from build123d import *

# Parameters (mm, degrees)
F3_R     = 2.291344539
F4_DEPTH = 2.5
F5_R     = 2.75
F6_DEPTH = 1


with BuildPart() as f1:
    # F0 (on Front) → F1 (revolve)
    with BuildSketch(Plane.XZ):
        with BuildLine():
            Line((-6, 0), (0, 0))
            Line((0, 0), (0, 12))
            add(Edge.make_bspline(
                [(0, 12), (-3.2266811418, 11.7082983458), (-6.2449243477, 6.1923159091), (-6.0526283931, 3.414490179), (-6, 0)],
                knots=[0, 0, 0, 0, 0.5139326164, 1, 1, 1, 1], degree=3))
        make_face()
    revolve(axis=Axis((0, 0, 6), (0, 0, 1)))

    # F3 (on offset) → F4 (join, symmetric)
    with BuildSketch(Plane.XY.offset(12)):
        Circle(F3_R)
    extrude(amount=F4_DEPTH, both=True)

    # F5 (on face) → F6 (join)
    with BuildSketch(Plane.XY.offset(14.5)):
        Circle(F5_R)
    extrude(amount=F6_DEPTH)


solid = f1.part
Can you work these out from the model? Positions are in its coordinate system, mm. Round coordinates to 2 decimals unless told otherwise and drop trailing zeros. Write each loop counter-clockwise with the first axis right and the second up, starting at its lowest first coordinate (ties: lowest second). Pieces come first, ordered by that corner, then holes. Notation, with made-up numbers: (-30.5, -8) -> (-13.5, -8) arc R8 cw to (-13.5, 2) -> close; hole circle Ø1 at (68.25, -11). An arc over 180 degrees is marked (long way). Use one line per item in the form item = value. Start each with the question number.
Q1. Imagine slicing it at A-A (z = 13). Please give me the cut outline in (x, y).
Q2. I'm going to push flat-ended pins straight in: P1, Ø3, axis at x = -2.5, y = -3.5, coming from the +Z side; P2, Ø4, axis at x = -4.5, y = 3.5, coming from the +Z side; P3, Ø4, axis at y = 1, z = 14, coming from the +X side. Where does each tip first touch, or does it pass through?
Q3. We'd pull the mould along Z, two halves only. Please class faces 1 (the face through (-0.596, -2.685, 14.993)), 2 (the face through (-2.29, 0.1, 12.9)), 3 (the face through (0, 0, 0)): +Z half, -Z half, draft (parallel to the pull), parting line (faces both ways), or undercut.
Q4. If I drill on probe 1 along X at (y, z) = (-0.5, 3.5); probe 2 along X at (y, z) = (1.75, 5.75); probe 3 along Z at (x, y) = (-4, -3.5), over which ranges is the centre line in solid material (lowest first)? Write a range as [from, to].
Worked out:
q1.outline = circle Ø4.58 at (0, 0)
q2.P1 = 10.9
q2.P2 = 10.05
q2.P3 = 2.75
q3.face_1 = draft
q3.face_2 = undercut
q3.face_3 = -Z half
q4.probe_1 = [-6.01, 6.01]
q4.probe_2 = [-5.49, 5.49]
q4.probe_3 = [0, 7.23]
